Work out the finished part from the listing and answer in its coordinate system (mm). Face numbers are marked on the shaded views. A direction names the side the tool comes from. Give positions to 0.01 mm unless a question says otherwise; leave off trailing zeros. Order: outer loops, then holes, each group sorted by start corner. A loop starts at its lowest first (then second) coordinate and runs counter-clockwise, first axis right, second up. Notation, with made-up numbers: (27, 43.5) - (79, 43.5) arc R19 ccw to (79, 63.5) - close; hole circle Ø6 at (24.25, 54). An arc over 180 degrees is marked (long way). Write each question's results on one line, items separated by ' | '.
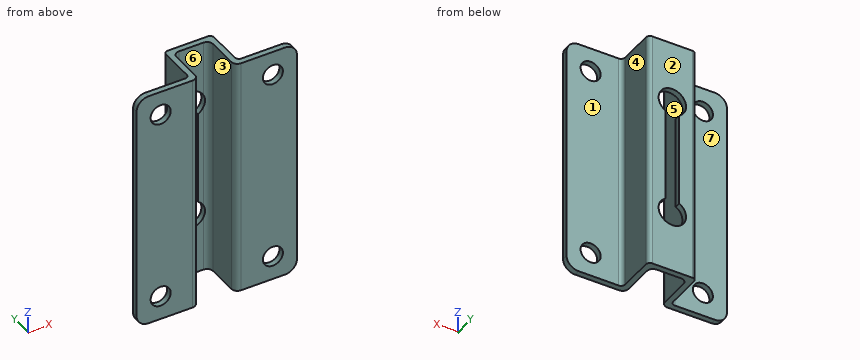
Autodesk Inventor part; units mm, degrees
ref_plane "YZ Plane" through (0, 0, 0) normal (1, 0, 0) x (0, 1, 0)
ref_plane "XZ Plane" through (0, 0, 0) normal (0, 1, 0) x (-1, 0, 0)
ref_plane "XY Plane" through (0, 0, 0) normal (0, 0, 1) x (1, 0, 0)
sketch "Sketch1" plane through (0, 0, 0) normal (0, 1, 0) x (-1, 0, 0)
  line L0 (-20, 30) -> (20, 30)
  line L1 (20, 30) -> (20, -30)
  line L2 (20, -30) -> (-20, -30)
  line L3 (-20, -30) -> (-20, 30)
  line L4 (-20, 30) -> (20, -30) construction
  line L5 (20, 30) -> (-20, -30) construction
  point P0 (0, 0)
  dimension "d0" = 40
  dimension "d1" = 60
extrude "Extrusion1" add sketch "Sketch1" along normal blind 12
sketch "Sketch2" plane through (-20, 0, 30) normal (0, 0, 1) x (1, 0, 0)
  line L0 (0, 0) -> (0, 12)
  line L1 (0, 0) -> (0, 1.45)
  line L2 (0, 1.45) -> (14, 1.45)
  line L3 (14, 1.45) -> (14, 12)
  line L4 (40, 12) -> (0, 12)
  line L5 (14, 12) -> (26, 12)
  line L6 (26, 12) -> (26, 1.45)
  line L7 (26, 1.45) -> (40, 1.45)
  line L8 (40, 0) -> (40, 12)
  line L9 (0, 12) -> (14, 12)
  line L10 (14, 12) -> (14, 1.45)
  line L11 (14, 1.45) -> (0, 1.45)
  line L12 (0, 1.45) -> (0, 12)
  line L13 (26, 1.45) -> (40, 1.45)
  line L14 (40, 1.45) -> (40, 12)
  line L15 (40, 12) -> (26, 12)
  line L16 (26, 12) -> (26, 1.45)
  line L17 (14, 1.45) -> (15.45, 1.45)
  line L18 (15.45, 1.45) -> (15.45, 12)
  line L19 (14, 12) -> (14, 10.55)
  line L20 (14, 10.55) -> (26, 10.55)
  line L21 (26, 12) -> (24.55, 12)
  line L22 (24.55, 12) -> (24.55, 1.45)
  line L23 (15.45, 10.55) -> (24.55, 10.55)
  line L24 (24.55, 10.55) -> (24.55, 0)
  line L25 (24.55, 0) -> (15.45, 0)
  line L26 (15.45, 0) -> (15.45, 10.55)
  point P0 (20, 0)
  point P1 (24.55, 1.45)
  point P2 (24.55, 10.55)
  point P3 (15.45, 1.45)
  dimension "d4" = 1.45
  dimension "d5" = 14
  dimension "d6" = 12
  dimension "d10" = 1.45
  dimension "d11" = 1.45
  dimension "d12" = 1.45
extrude "Extrusion2" cut sketch "Sketch2" against normal up to surface (60 mm away) contours L0 L4 L3 L2 | L18 L20 L22 L24 L25 L26 | L4 L8 L7 L6
sketch "Sketch3" plane through (-6, 1.45, 30) normal (0, 1, 0) x (1, 0, 0)
  line L0 (-14, 60) -> (-14, 0)
  line L1 (26, 0) -> (26, 60)
  line L2 (-14, 60) -> (26, 60)
  line L3 (26, 60) -> (26, 0)
  line L4 (26, 0) -> (-14, 0)
  line L5 (-14, 0) -> (-14, 60)
  line L6 (-14, 60) -> (-8, 60)
  line L7 (-8, 60) -> (-8, 54)
  line L8 (-8, 54) -> (-14, 54)
  line L9 (-14, 54) -> (-14, 60)
  circle A0 centre (-8, 54) radius 2.5
  line L10 (26, 60) -> (20, 60)
  line L11 (20, 60) -> (20, 54)
  line L12 (20, 54) -> (26, 54)
  line L13 (26, 54) -> (26, 60)
  circle A1 centre (20, 54) radius 2.5
  line L14 (26, 0) -> (25.5, 0)
  line L15 (26, 0) -> (20, 0)
  line L16 (20, 0) -> (20, 6)
  line L17 (20, 6) -> (26, 6)
  line L18 (26, 6) -> (26, 0)
  line L19 (-14, 0) -> (-8, 0)
  line L20 (-8, 0) -> (-8, 6)
  line L21 (-8, 6) -> (-14, 6)
  line L22 (-14, 6) -> (-14, 0)
  circle A2 centre (-8, 6) radius 2.5
  circle A3 centre (20, 6) radius 2.5
  point P0 (6, 30)
  dimension "d15" = 6
  dimension "d16" = 6
  dimension "d17" = 5
  dimension "d18" = 6
  dimension "d19" = 6
  dimension "d20" = 5
  dimension "d21" = 6
  dimension "d22" = 6
  dimension "d23" = 5
  dimension "d24" = 5
  dimension "d25" = 6
  dimension "d26" = 6
extrude "Extrusion3" cut sketch "Sketch3" against normal blind 12 contours A0 L7 L8 | L8 L7 A0 | A2 L20 L21 | L21 L20 A2 | A1 L12 L11 | L11 L12 A1 | A3 L17 L16 | L16 L17 A3
sketch "Sketch4" plane through (0, 12, 0) normal (0, 1, 0) x (1, 0, 0)
  line L0 (4.55, 30) -> (-4.55, 30)
  line L1 (0, 30) -> (0, 18)
  line L2 (-4.55, -30) -> (4.55, -30)
  line L3 (0, -30) -> (0, -18)
  line L4 (0, 18) -> (0, 14.575)
  line L5 (0, -18) -> (0, -14.575)
  circle A0 centre (0, 14.575) radius 3.425
  circle A1 centre (0, -14.575) radius 3.425
  line L6 (0, 14.575) -> (1.7125, 14.575)
  line L7 (1.7125, 14.575) -> (1.7125, -14.575)
  line L8 (1.7125, -14.575) -> (0, -14.575)
  line L9 (0, -14.575) -> (0, 14.575)
  line L10 (0, 14.575) -> (1.7125, 14.575) construction
  line L11 (0, -14.575) -> (-1.7125, -14.575)
  line L12 (-1.7125, -14.575) -> (-1.7125, 14.575)
  line L13 (-1.7125, 14.575) -> (0, 14.575)
  line L14 (0, 14.575) -> (0, -14.575)
  point P0 (0, 0)
  point P1 (3.55, 30)
  point P2 (-3.55, 30)
  point P3 (-3.55, -30)
  point P4 (3.55, -30)
  point P5 (1.7125, -11.6089)
  point P6 (1.7125, 11.6089)
  point P7 (-1.7125, 11.6089)
  point P8 (-1.7125, -11.6089)
  dimension "d29" = 12
  dimension "d30" = 12
  dimension "d31" = 3.425
  dimension "d32" = 3.425
  dimension "d33" = 1.7125
  dimension "d34" = 0
  dimension "d35" = 1.7125
extrude "Extrusion4" cut sketch "Sketch4" against normal blind 12
fillet "Fillet3" radius 3 4 edges at (20, 0.725, 30) (-20, 0.725, 30) (20, 0.725, -30) (-20, 0.725, -30)
fillet "Fillet4" radius 1 4 edges at (6, 1.45, 0) (6, 12, 0) (-6, 12, 0) (-6, 1.45, 0)
fillet "Fillet4" radius 1.5 4 edges at (-4.55, 10.55, 0) (4.55, 10.55, 0) (4.55, 0, 0) (-4.55, 0, 0)
equation "\"d10\" = d4"
equation "\"d11\" = d4"
equation "\"d12\" = d4"
equation "\"d18\" = d15"
equation "\"d19\" = d16"
equation "\"d20\" = d17"
equation "\"d21\" = d15"
equation "\"d22\" = d16"
equation "\"d23\" = d17"
equation "\"d24\" = d17"
equation "\"d25\" = d15"
equation "\"d26\" = d16"
equation "\"d30\" = d29"
equation "\"d32\" = d31"
properties part number "part1pasador"
1. Determine the mould class of the marked faces 4, 5, 6 and 7 for opening direction X: +X half, -X half, draft (parallel to the pull), parting line (faces both ways), or undercut.
Answer list:
face 4: +X half | face 5: undercut | face 6: undercut | face 7: draft
2. A cutting plane is placed at D-D, the plane x = 14. Write down the section's boundary in (y, z).
Answer list:
outline: (0, -30) - (1.45, -30) - (1.45, -26.5) - (0, -26.5) - close; (0, -21.5) - (1.45, -21.5) - (1.45, 21.5) - (0, 21.5) - close; (0, 26.5) - (1.45, 26.5) - (1.45, 30) - (0, 30) - close
3. Straight lines are drawn through the part: line 1 (Z direction, x = 14, y = 0.9); line 2 (X direction, y = 0.85, z = -24); line 3 (X direction, y = 0.75, z = 24). For each, find the intervals that lie inside material, in ascending order. Write a range as [from, to].
Answer list:
line 1: [-30, -26.5], [-21.5, 21.5], [26.5, 30] | line 2: [-20, -16.5], [-11.5, -4.7], [4.7, 11.5], [16.5, 20] | line 3: [-20, -16.5], [-11.5, -4.75], [4.75, 11.5], [16.5, 20]
4. A cutting plane is placed at A-A, the plane z = -8. Write down the section's boundary in (x, y).
Answer list:
outline: (-20, 0) - (-6.05, 0) arc R1.5 ccw to (-4.55, 1.5) - (-4.55, 9.05) arc R1.5 cw to (-3.05, 10.55) - (-1.71, 10.55) - (-1.71, 12) - (-5, 12) arc R1 ccw to (-6, 11) - (-6, 2.45) arc R1 cw to (-7, 1.45) - (-20, 1.45) - close; (1.71, 10.55) - (3.05, 10.55) arc R1.5 cw to (4.55, 9.05) - (4.55, 1.5) arc R1.5 ccw to (6.05, 0) - (20, 0) - (20, 1.45) - (7, 1.45) arc R1 cw to (6, 2.45) - (6, 11) arc R1 ccw to (5, 12) - (1.71, 12) - close
5. Given P1, Ø1.2, axis at y = 11, z = 1.5, coming from the -X side; P2, Ø3, axis at x = -1.5, z = -21.5, coming from the -Y side; P3, Ø1.5, axis at x = 2.5, z = -5.5, coming from the -Y side, each flat-ended and moving along its own axis, determine where each tip first touches the part or whether it passes through.
Answer list:
P1: x = -6 | P2: y = 10.55 | P3: y = 10.54
6. A cutting plane is placed at B-B, the plane y = 6. Write down the section's boundary in (x, z).
Answer list:
outline: (-6, -30) - (-4.55, -30) - (-4.55, 30) - (-6, 30) - close; (4.55, -30) - (6, -30) - (6, 30) - (4.55, 30) - close
7. A cutting plane is placed at C-C, the plane z = -24. Write down the section's boundary in (x, y), then the cut area to 3 significant figures.
Answer list:
outline: (-20, 0) - (-16.5, 0) - (-16.5, 1.45) - (-20, 1.45) - close; (-11.5, 0) - (-6.05, 0) arc R1.5 ccw to (-4.55, 1.5) - (-4.55, 9.05) arc R1.5 cw to (-3.05, 10.55) - (3.05, 10.55) arc R1.5 cw to (4.55, 9.05) - (4.55, 1.5) arc R1.5 ccw to (6.05, 0) - (11.5, 0) - (11.5, 1.45) - (7, 1.45) arc R1 cw to (6, 2.45) - (6, 11) arc R1 ccw to (5, 12) - (-5, 12) arc R1 ccw to (-6, 11) - (-6, 2.45) arc R1 cw to (-7, 1.45) - (-11.5, 1.45) - close; (16.5, 0) - (20, 0) - (20, 1.45) - (16.5, 1.45) - close | area: 74.1 mm^2
8. A tool of negligible diameter and unlimited length cuts with its end or side. For the marked faces 1, 2 and 3, from which of +Z, -Z, +X, -X, +Y, -Y can it reach the whole face along a straight path? Write none if from no direction.
Answer list:
face 1: +Z, -Z, +X, +Y | face 2: +Z, -Z, +X, -X, +Y | face 3: +Z, -Z, -Y
